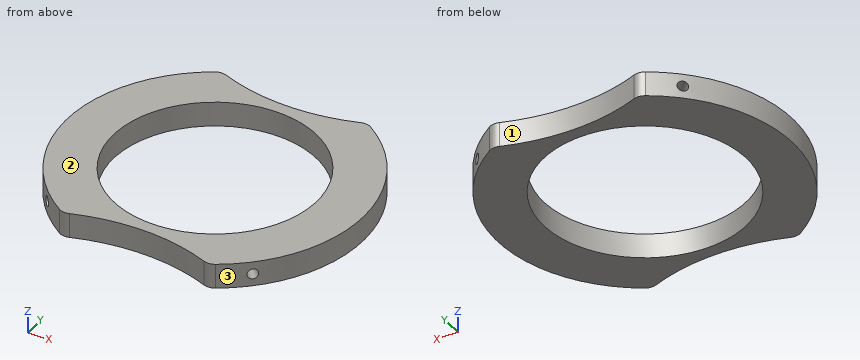
Autodesk Inventor part; units mm, degrees
ref_plane "Work Plane4" through (26.9408, -26.9408, 0) normal (-0.7071, 0.7071, 0) x (0, 0, 1)
ref_plane "XY Plane" through (0, 0, 0) normal (0, 0, 1) x (1, 0, 0)
ref_plane "Work Plane1" through (0, 38.1, 0) normal (0, 1, 0) x (-1, 0, 0)
sketch "Sketch1" plane through (0, 0, 0) normal (0, 0, 1) x (1, 0, 0)
  circle A0 centre (0, 0) radius 38.1
  arc A1 (-19.05, 32.9956) -> (19.05, 32.9956) centre (0, 80.0884) ccw
  line L0 (-38.1, 0) -> (38.1, 0) construction
  arc A2 (19.05, -32.9956) -> (-19.05, -32.9956) centre (0, -80.0884) ccw
  circle A3 centre (0, 0) radius 26.1134
  line L1 (0, 29.2884) -> (0, 26.1134) construction
  point P0 (-19.05, -32.9956)
  point P1 (19.05, -32.9956)
  dimension "d0" = 76.2
  dimension "d1" = 38.1
  dimension "d3" = 50.8
  dimension "d4" = 3.175
extrude "Extrusion1" add sketch "Sketch1" along normal mid plane 6.35 contours A0 A2 A1
ref_plane "Work Plane4" through (26.9408, -26.9408, 0) normal (-0.7071, 0.7071, 0) x (0, 0, 1)
ref_plane "Work Plane3" through (38.1, 38.1, 0) normal (-0.7071, 0.7071, 0) x (0, 0, 1)
sketch "Sketch2" plane through (26.9408, -26.9408, 0) normal (-0.7071, 0.7071, 0) x (0, 0, 1)
  point P0 (0, 0)
  point P1 (0, 0)
hole "Hole1" at (26.9408, -26.9408, 0) direction (-0.7071, 0.7071, 0) diameter 2.6416 depth 6.35 tip angle 118
pattern_circular "Circular Pattern1" count 4 over 360 about axis through (0, 0, 0) along (0, 0, 1) of "Hole1"
fillet "Fillet1" radius 3.175 4 edges at (-19.05, -32.9956, 0) (19.05, -32.9956, 0) (19.05, 32.9956, 0) (-19.05, 32.9956, 0)
ref_plane "Work Plane1" through (0, 38.1, 0) normal (0, 1, 0) x (-1, 0, 0)
ref_plane "Work Plane2" through (38.1, 0, 0) normal (1, 0, 0) x (0, 1, 0)
properties part number "ShockCordSupportBulkhead"
Source: CAD feature listing. Evaluate the final solid. Frame: model axes, mm. Face numbers are marked on the shaded views. Give positions to 0.01 mm unless a question says otherwise; leave off trailing zeros. Order: outer loops, then holes, each group sorted by start corner. A loop starts at its lowest first (then second) coordinate and runs counter-clockwise, first axis right, second up. Notation, with made-up numbers: (-31.75, 56.5) -> (-6.75, 56.5) arc R12 ccw to (-6.75, 60.5) -> close; hole circle Ø7 at (89, 51). An arc over 180 degrees is marked (long way). Use a Markdown table: item, result.
1) Mould query, pull axis X, two halves, no side actions, for the marked faces 1, 2 and 3. Classes: +X half, -X half, draft (parallel to the pull), parting line (faces both ways), or undercut.
Answer list:
| item | result |
|---|---|
| face 1 | undercut |
| face 2 | draft |
| face 3 | +X half |
2) Section query C-C, the plane x = 33. Return the cut outline in (y, z) (3 decimals), then the cut area to 3 significant figures.
Answer list:
| item | result |
|---|---|
| outline | (-19.042, -3.175) -> (19.042, -3.175) -> (19.042, 3.175) -> (-19.042, 3.175) -> close |
| area | 242 mm² |
3) Section query A-A, the plane y = 0. Return the cut outline in (x, z) (3 decimals), then the cut area to 3 significant figures.
Answer list:
| item | result |
|---|---|
| outline | (-38.1, -3.175) -> (-26.113, -3.175) -> (-26.113, 3.175) -> (-38.1, 3.175) -> close; (26.113, -3.175) -> (38.1, -3.175) -> (38.1, 3.175) -> (26.113, 3.175) -> close |
| area | 152 mm² |
4) Contact query for flat-ended pins moving along their axis: P1, Ø1, axis at x = 22, z = -1, coming from the -Y side; P2, Ø1.5, axis at y = -18.5, z = 1.5, coming from the -X side; P3, Ø1, axis at y = 3.5, z = 1, coming from the +X side. Output: stop coordinate, or through.
Answer list:
| item | result |
|---|---|
| P1 | y = -31.45 |
| P2 | x = -33.71 |
| P3 | x = 37.98 |
5) Section query B-B, the plane x = 0. Return the cut outline in (y, z) (3 decimals).
Answer list:
| item | result |
|---|---|
| outline | (-29.288, -3.175) -> (-26.113, -3.175) -> (-26.113, 3.175) -> (-29.288, 3.175) -> close; (26.113, -3.175) -> (29.288, -3.175) -> (29.288, 3.175) -> (26.113, 3.175) -> close |
6) Ray query, line 1 along Y through (x, z) = (20, -1.75); line 2 along Y through (x, z) = (12, 0.5); line 3 along X through (y, z) = (19.5, -2.5). Return the intervals inside material, ascending. Write a range as [from, to].
Answer list:
| item | result |
|---|---|
| line 1 | [-32.39, -16.79], [16.79, 32.39] |
| line 2 | [-30.73, -23.19], [23.19, 30.73] |
| line 3 | [-32.73, -17.37], [17.37, 32.73] |
